```python
from build123d import *

# Parameters (mm, degrees)
BOSS_EXTRUDE1_DEPTH = 6.35
CUT_EXTRUDE1_REACH  = 22.016
SKETCH2_R           = 1.7
SKETCH2_R_2         = 1.45


with BuildPart() as part:
    # Sketch1 → Boss-Extrude1 (new body)
    with BuildSketch(Plane.XY):
        with BuildLine():
            Line((515.21, 42.790633073), (512.71, 42.790633073))
            Line((512.71, 42.790633073), (512.71, 48.790633073))
            Line((512.71, 48.790633073), (502.194313483, 48.790633073))
            ThreePointArc((502.194313483, 48.790633073), (495.194313483, 55.790633073), (502.194313483, 62.790633073))
            Line((502.194313483, 62.790633073), (512.71, 62.790633073))
            Line((512.71, 62.790633073), (512.71, 68.790633073))
            Line((512.71, 68.790633073), (515.21, 68.790633073))
            Line((515.21, 68.790633073), (515.21, 42.790633073))
        make_face()
        with BuildLine():
            Line((511.694313483, 53.540633073), (499.21, 53.540633073))
            ThreePointArc((499.21, 53.540633073), (498.194313483, 55.790633073), (499.21, 58.040633073))
            Line((499.21, 58.040633073), (511.694313483, 58.040633073))
            ThreePointArc((511.694313483, 58.040633073), (512.71, 55.790633073), (511.694313483, 53.540633073))
        make_face(mode=Mode.SUBTRACT)
    extrude(amount=BOSS_EXTRUDE1_DEPTH)

    # Sketch2 → Cut-Extrude1 (cut, up to next)
    with BuildSketch(Plane(origin=(515.21, 0, 0), x_dir=(0, 0, -1), z_dir=(1, 0, 0)), mode=Mode.PRIVATE) as cut_extrude1_sk1:
        with Locations((-3.175, 45.790633073)):
            Circle(SKETCH2_R)
    cut_extrude1_tool1 = extrude(cut_extrude1_sk1.sketch, amount=-CUT_EXTRUDE1_REACH, mode=Mode.PRIVATE) & part.part
    add(cut_extrude1_tool1.solids().sort_by_distance((515.21, 45.790633, 3.175))[0], mode=Mode.SUBTRACT)
    # Sketch2 → Cut-Extrude1 (cut, up to next)
    with BuildSketch(Plane(origin=(515.21, 0, 0), x_dir=(0, 0, -1), z_dir=(1, 0, 0)), mode=Mode.PRIVATE) as cut_extrude1_sk2:
        with Locations((-3.35, 55.790633073)):
            Circle(SKETCH2_R_2)
    cut_extrude1_tool2 = extrude(cut_extrude1_sk2.sketch, amount=-CUT_EXTRUDE1_REACH, mode=Mode.PRIVATE) & part.part
    add(cut_extrude1_tool2.solids().sort_by_distance((515.21, 55.790633, 3.35))[0], mode=Mode.SUBTRACT)
    # Sketch2 → Cut-Extrude1 (cut, up to next)
    with BuildSketch(Plane(origin=(515.21, 0, 0), x_dir=(0, 0, -1), z_dir=(1, 0, 0)), mode=Mode.PRIVATE) as cut_extrude1_sk3:
        with Locations((-3.175, 65.790633073)):
            Circle(SKETCH2_R)
    cut_extrude1_tool3 = extrude(cut_extrude1_sk3.sketch, amount=-CUT_EXTRUDE1_REACH, mode=Mode.PRIVATE) & part.part
    add(cut_extrude1_tool3.solids().sort_by_distance((515.21, 65.790633, 3.175))[0], mode=Mode.SUBTRACT)


solid = part.part
```
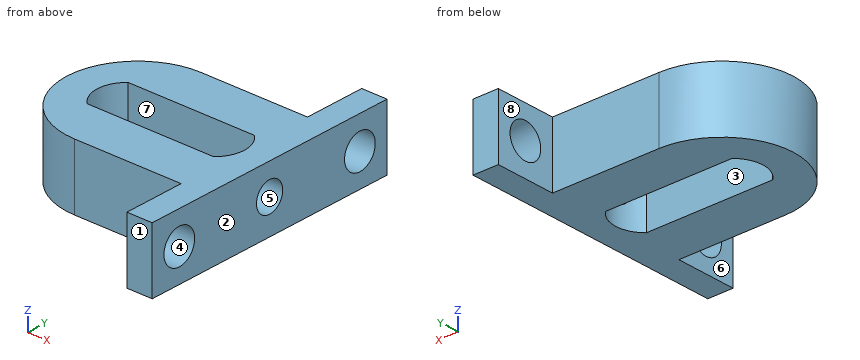
Verification items for the finished model (mm, model axes). Face numbers are marked on the shaded views. A direction names the side the tool comes from. Give positions to 0.01 mm unless a question says otherwise; leave off trailing zeros. Loops run counter-clockwise (first coordinate to the right, second up) from the corner with the lowest first, then second, coordinate; pieces in that order, holes last. Notation, with made-up numbers: M 75.5,27 L 86.5,27 A23 ccw 86.5,53 Z; hole C 22,26.25 d4. An arc over 180 degrees is marked long. One line per question, with ' | ' between items.
Item 1: Section check D-D, the plane z = 2.75. Record the cut outline in (x, y).
Completed:
outline: M 499.21,53.54 A3 cw 499.21,58.04 L 511.69,58.04 A3 cw 512.4,57.11 L 515.21,57.11 L 515.21,64.14 L 512.71,64.14 L 512.71,62.79 L 502.19,62.79 A7 ccw 502.19,48.79 L 512.71,48.79 L 512.71,47.44 L 515.21,47.44 L 515.21,54.47 L 512.4,54.47 A3 cw 511.69,53.54 Z; M 512.71,42.79 L 515.21,42.79 L 515.21,44.14 L 512.71,44.14 Z; M 512.71,67.44 L 515.21,67.44 L 515.21,68.79 L 512.71,68.79 Z
Item 2: Tool access check on the marked faces 5, 6, 7 and 8. Record the directions out of +Z, -Z, +X, -X, +Y, -Y that give a thin tool (end or side, any length) a straight path to the whole face; none if there is none.
Completed:
face 5: +X | face 6: +Z, -Z, -X, -Y | face 7: +Z, -Z | face 8: +Z, -Z, -X, +Y
Item 3: Thickness scan on line 1 (Y direction, x = 504.5, z = 2.5); line 2 (X direction, y = 45.25, z = 1.5); line 3 (Y direction, x = 513.15, z = 3.35). Record the ranges inside material, lowest first. Write a range as [from, to].
Completed:
line 1: y = [48.79, 53.54], [58.04, 62.79] | line 2: x = [512.71, 515.21] | line 3: y = [42.79, 44.1], [47.48, 54.34], [57.24, 64.1], [67.48, 68.79]
Item 4: Depth check by flat-ended pin: P1, Ø3, axis at x = 498.5, y = 64, coming from the +Z side; P2, Ø1.5, axis at x = 499, z = 1, coming from the -Y side; P3, Ø1.8, axis at y = 64.5, z = 3.5, coming from the -X side; P4, Ø3, axis at x = 506.5, z = 4, coming from the +Y side. Enter the tip coordinate at first touch or a pass-through.
Completed:
P1: passes through | P2: stops at y = 49.23 | P3: stops at x = 512.71 | P4: stops at y = 62.79
Item 5: Section check C-C, the plane y = 64.5. Record the cut outline in (x, z), plus the area to 3 significant figures.
Completed:
outline: M 512.71,0 L 515.21,0 L 515.21,2.07 L 512.71,2.07 Z; M 512.71,4.28 L 515.21,4.28 L 515.21,6.35 L 512.71,6.35 Z | area: 10.3 mm^2
Item 6: Section check B-B, the plane z = 0.5. Record the cut outline in (x, y).
Completed:
outline: M 502.19,48.79 L 512.71,48.79 L 512.71,42.79 L 515.21,42.79 L 515.21,68.79 L 512.71,68.79 L 512.71,62.79 L 502.19,62.79 A7 ccw Z; hole M 499.21,53.54 L 511.69,53.54 A3 ccw 511.69,58.04 L 499.21,58.04 A3 ccw Z
Item 7: Section check A-A, the plane x = 508.5. Record the cut outline in (y, z).
Completed:
outline: M 48.79,0 L 53.54,0 L 53.54,6.35 L 48.79,6.35 Z; M 58.04,0 L 62.79,0 L 62.79,6.35 L 58.04,6.35 Z
Item 8: Draft check along Y on the marked faces 1, 2, 3 and 4. Enter one of: +Y half, -Y half, draft (parallel to the pull), parting line (faces both ways), or undercut.
Completed:
face 1: -Y half | face 2: draft | face 3: undercut | face 4: undercut
